Design review of the part shown in the three views and the two pictorial views. Dimensions are in mm from the part's minimum x, y and z. Round coordinates to 2 decimals unless told otherwise and drop trailing zeros. Order: outer loops, then holes, each group sorted by start corner. A loop starts at its lowest first (then second) coordinate and runs counter-clockwise, first axis right, second up. Notation, with made-up numbers: M 32,78.25 L 83,78.25 A26 cw 83,96.25 Z; hole C 15,10 d5. An arc over 180 degrees is marked long. Write each question's results on one line, items separated by ' | '. Start each with the question number.
Item 1: The part is to be moulded in two halves that separate along Z. For the marked faces 1, 2, 3 and 4, say which applies: +Z half, -Z half, draft (parallel to the pull), parting line (faces both ways), or undercut.
Item 2: Take a section at C-C, the plane x = 60.96. Write out the cut boundary in (y, z), plus the area to 3 significant figures.
Item 3: Wall thickness on line 1 (X direction, y = 1.25, z = 4.75); line 2 (X direction, y = 3.25, z = 5.25); line 3 (Z direction, x = 60.96, y = 3.5): over which ranges is each line inside the solid? List them lowest first. Write a range as [from, to].
Item 4: Take a section at D-D, the plane z = 8. Write out the cut boundary in (x, y).
Item 5: Take a section at A-A, the plane y = 4. Write out the cut boundary in (x, z) (3 decimals).
Item 6: Take a section at B-B, the plane z = 4. Write out the cut boundary in (x, y), plus the area to 3 significant figures.
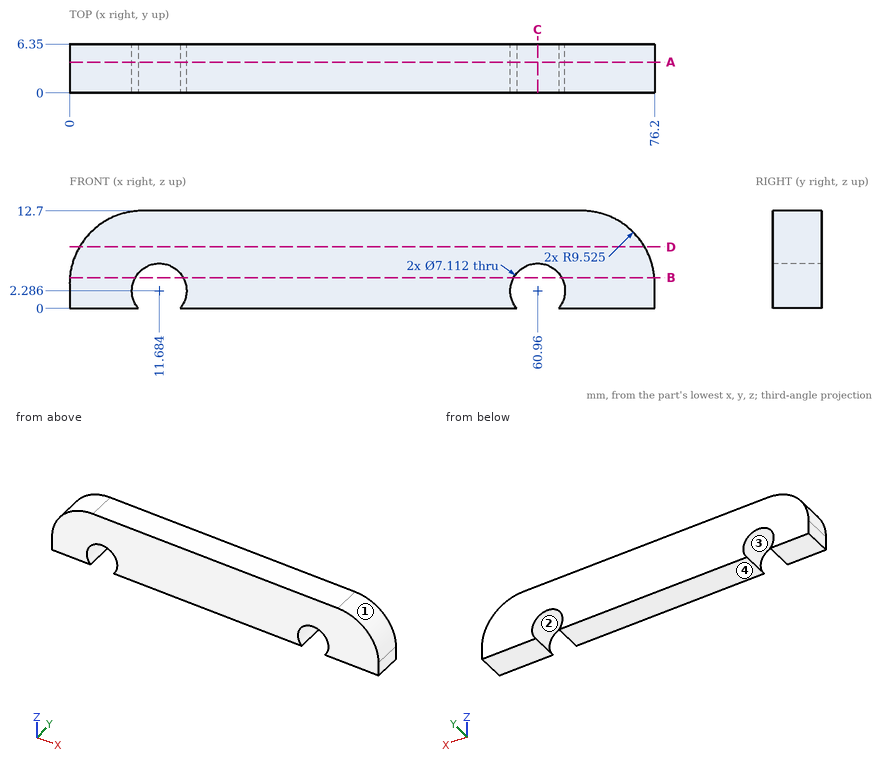
Results list:
1) face 1: +Z half | face 2: undercut | face 3: undercut | face 4: -Z half
2) outline: M 0,5.84 L 6.35,5.84 L 6.35,12.7 L 0,12.7 Z | area: 43.5 mm²
3) line 1: [0.13, 9.12], [14.25, 58.4], [63.52, 76.07] | line 2: [0.23, 9.72], [13.65, 59], [62.92, 75.97] | line 3: [5.84, 12.7]
4) outline: M 1.31,0 L 74.89,0 L 74.89,6.35 L 1.31,6.35 Z
5) outline: M 0,0 L 8.96,0 A3.556 cw long 14.408,0 L 58.236,0 A3.556 cw long 63.684,0 L 76.2,0 L 76.2,3.175 A9.525 ccw 66.675,12.7 L 9.525,12.7 A9.525 ccw 0,3.175 Z
6) outline: M 0.04,0 L 8.57,0 L 8.57,6.35 L 0.04,6.35 Z; M 14.8,0 L 57.84,0 L 57.84,6.35 L 14.8,6.35 Z; M 64.08,0 L 76.16,0 L 76.16,6.35 L 64.08,6.35 Z | area: 404 mm²
